Build history of the part. All positions in model axes, mm. A direction names the side the tool comes from. Round coordinates to 2 decimals unless told otherwise and drop trailing zeros. Order: outer loops, then holes, each group sorted by start corner. A loop starts at its lowest first (then second) coordinate and runs counter-clockwise, first axis right, second up. Notation, with made-up numbers: (82, 51.25) -> (124, 51.25) arc R16 ccw to (124, 62.25) -> close; hole circle Ø10 at (6, -24.75). An arc over 180 degrees is marked (long way). Use a Markdown table: item, result. Add a question column.
Item 1: Two-plate mould, pull along X, no slides. Class faces 1 (the face through (18, 4, 4)), 2 (the face through (23, 0, -6)), 3 (the face through (28, -0.1, 3.3)): released by +X, released by -X, zero draft, split by the parting line, or undercut.
Item 2: Slice it at B-B, the plane x = 123. Give the cut face in (y, z), plus the area to 3 significant figures.
Item 3: 3-axis set-ups, long thin cutter, end or side, ignore diameter. For faces 4 (the face through (18.76, 4.88, -1.08)), 5 (the face through (3.03, 9.76, -2.17)), 6 (the face through (16.028, -8.923, -1.172)): which of +Z, -Z, +X, -X, +Y, -Y reach the whole face in a straight line?
Item 4: Pin check, flat tips, straight feed: pin 1 (12 mm diameter, centred on y = 8, z = -4.5, fed in from +X); pin 2 (2 mm diameter, centred on x = 132, z = 0.5, fed in from +Y); pin 3 (4 mm diameter, centred on x = 52.5, z = 3.5, fed in from -Y). Stop position of each tip, or through.
Item 5: Slice it at A-A, the plane x = 62. Give the cut face in (y, z), plus the area to 3 significant figures.
Item 6: Probe L1, parallel to Z at x = 11, y = -5.5; L2, parallel to X at y = 1.75, z = 8.75; L3, parallel to Y at x = 132, z = 0.25. List the from-to ranges inside material, lowest first.
Autodesk Inventor part; units mm, degrees
ref_plane "工作平面1" through (98, 0, 0) normal (1, 0, 0) x (0, 0, -1)
ref_plane "工作平面2" through (68, 0, 0) normal (1, 0, 0) x (0, 0, -1)
ref_plane "YZ Plane" through (0, 0, 0) normal (1, 0, 0) x (0, 1, 0)
sketch "草图1" plane through (0, 0, 0) normal (0, 1, 0) x (-1, 0, 0)
  line L0 (0, 0) -> (0, 9)
  line L1 (0, 9) -> (-1, 10)
  line L2 (-1, 10) -> (-5, 10)
  line L3 (-5, 10) -> (-6, 9)
  line L4 (29.6, 0) -> (-177.6, 0)
  arc A0 (-14, 9) -> (-6, 9) centre (-10, 13) ccw
  line L5 (-14, 9) -> (-18, 9)
  line L6 (-18, 9) -> (-18, 5)
  line L7 (-18, 5) -> (-19.5, 5)
  line L8 (-19.5, 5) -> (-19.5, 6)
  line L9 (-19.5, 6) -> (-27, 6)
  line L10 (-27, 6) -> (-28, 5)
  line L11 (-28, 5) -> (-28, 3)
  line L12 (-28, 3) -> (-147, 3)
  line L13 (0, 0) -> (-118, 0)
  line L14 (-147, 3) -> (-148, 2)
  line L15 (-148, 2) -> (-148, 0)
  dimension "d0" = 10
  dimension "d4" = 45
  dimension "d5" = 1
  dimension "d6" = 45
  dimension "d7" = 1
  dimension "d8" = 6
  dimension "d9" = 6
  dimension "d10" = 45
  dimension "d11" = 1
  dimension "d12" = 3
  dimension "d13" = 4
  dimension "d14" = 10
  dimension "d16" = 28
  dimension "d17" = 9
  dimension "d18" = 1.5
  dimension "d19" = 1
  dimension "d21" = 45
  dimension "d22" = 1
  dimension "d23" = 130
revolve "旋转1" add sketch "草图1" angle 360 about axis through (-10, 0, 0) along (1, 0, 0)
thread "螺纹1"
ref_plane "工作平面1" through (98, 0, 0) normal (1, 0, 0) x (0, 0, -1)
sketch "草图2" plane through (98, 0, 0) normal (1, 0, 0) x (0, 0, -1)
  circle A0 centre (0, 0) radius 2.9
  circle A1 centre (0, 0) radius 3
  dimension "d27" = 5.8
  dimension "d30" = 6
extrude "拉伸1" cut sketch "草图2" along normal through all
ref_plane "工作平面2" through (68, 0, 0) normal (1, 0, 0) x (0, 0, -1)
sketch "草图3" plane through (68, 0, 0) normal (1, 0, 0) x (0, 0, -1)
  circle A0 centre (0, 0) radius 2.95
  circle A1 centre (0, 0) radius 3
  dimension "d32" = 5.9
  dimension "d33" = 6
extrude "拉伸2" cut sketch "草图3" along normal through all
equation "\"d0\" = 0.5 * D"
equation "\"d8\" = b"
equation "\"d9\" = 0.5 * Md"
equation "\"d12\" = 0.5 * d3"
equation "\"d13\" = c_"
equation "\"d14\" = a"
equation "\"d16\" = h_"
equation "\"d23\" = L"
equation "\"d1\" = 4"
equation "\"d2\" = 12"
equation "\"d3\" = 6"
equation "\"h_\" = 28"
equation "\"a\" = 10"
equation "\"b\" = 6"
equation "\"c_\" = 4"
equation "\"D1\" = 16"
equation "\"Md\" = 12"
equation "\"L\" = 130"
properties part number "杆式油标" material "钢，软"
Check sheet entries:
| question | item | result |
|---|---|---|
| 1 | face 1 | undercut |
| 1 | face 2 | zero draft |
| 1 | face 3 | released by +X |
| 2 | outline | circle Ø5.8 at (0, 0) |
| 2 | area | 26.4 mm2 |
| 3 | face 4 | none |
| 3 | face 5 | +X, -X |
| 3 | face 6 | +X |
| 4 | pin 1 | x = 28 |
| 4 | pin 2 | y = 2.9 |
| 4 | pin 3 | y = -2.6 |
| 5 | outline | circle Ø6 at (0, 0) |
| 5 | area | 28.3 mm2 |
| 6 | L1 | -5 to 5 |
| 6 | L2 | 0 to 6.08, 13.92 to 18 |
| 6 | L3 | -2.89 to 2.89 |
